Here's how the part is built. I have some questions about the finished solid (model axes, mm). A direction names the side the tool comes from. Round coordinates to 2 decimals unless told otherwise and drop trailing zeros. Write each loop counter-clockwise with the first axis right and the second up, starting at its lowest first coordinate (ties: lowest second). Pieces come first, ordered by that corner, then holes. Notation, with made-up numbers: (14, 8) - (70, 8) arc R17 cw to (70, 14) - close; hole circle Ø1 at (21.25, 1.5). An arc over 180 degrees is marked (long way). One line per question, with ' | ' between items. Start each with the question number.
(1) If I drill on L1, parallel to Z at x = -10.5, y = 4.25; L2, parallel to X at y = -1, z = 5.25; L3, parallel to Y at x = 1.5, z = 4, over which ranges is the centre line in solid material (lowest first)?
(2) For faces 1 (the flat face through (5, -10, 2)), 2 (the cylindrical face through (0.54, -2.44, 3.55)), which set-ups out of +Z, -Z, +X, -X, +Y, -Y let a thin tool reach every point of the face, with its end or its side?
(3) Will these pins go through, and if not, where does the flat tip stop? pin 1 (1 mm diameter, centred on x = -3.5, z = 1, fed in from +Y); pin 2 (1 mm diameter, centred on x = 1, z = 3.5, fed in from -Y); pin 3 (2 mm diameter, centred on x = 7, y = 0, fed in from +Z); pin 4 (1 mm diameter, centred on y = 0.5, z = 4, fed in from -X).
(4) Thinking about a two-plate mould opening in X: for faces 3 (the cylindrical face through (-11.99, 0.53, 6.19)), 4 (the flat face through (-3, 0, 0)), 5 (the cylindrical face through (5.75, 0.05, 3.65)), which applies, pulls with the +X half, pulls with the -X half, needs draft (parallel to the pull), parting line crosses it, or undercut?
(5) Imagine slicing it at A-A (z = 3.25). Write out the boundary of the cut face in (x, y), plus the area to 3 significant figures.
from build123d import *

# Parameters (mm, degrees)
SKETCH_1_R          = 12
EXTRUDE_1_DEPTH     = 2
SKETCH_2_R          = 11
EXTRUDE_2_DEPTH     = 3.2
SKETCH_3_R          = 12
EXTRUDE_3_DEPTH     = 2
SKETCH_4_R          = 2.5
CUT_EXTRUDE_1_DEPTH = 30
SKETCH_3D_1_R       = 1.597010155
M3X0_5_1_D          = 2.5
M3X0_5_1_DEPTH      = 8.5
M3X0_5_1_TIP        = 0.751075774


with BuildPart() as part:
    # ｽｹｯﾁ1 → ﾎﾞｽ - 押し出し1 (new body)
    with BuildSketch(Plane.XY):
        Circle(SKETCH_1_R)
    extrude(amount=EXTRUDE_1_DEPTH)

    # ｽｹｯﾁ2 → ﾎﾞｽ - 押し出し2 (add)
    with BuildSketch(Plane.XY.offset(2)):
        Circle(SKETCH_2_R)
    extrude(amount=EXTRUDE_2_DEPTH)

    # ｽｹｯﾁ3 → ﾎﾞｽ - 押し出し3 (add)
    with BuildSketch(Plane.XY.offset(5.2)):
        Circle(SKETCH_3_R)
    extrude(amount=EXTRUDE_3_DEPTH)

    # ｽｹｯﾁ4 → ｶｯﾄ - 押し出し1 (cut)
    with BuildSketch(Plane(origin=(0, 0, 0), x_dir=(-1, 0, 0), z_dir=(0, 0, -1))):
        Circle(SKETCH_4_R)
    extrude(amount=-CUT_EXTRUDE_1_DEPTH, mode=Mode.SUBTRACT)

    # ｶｯﾄ - ｽｲｰﾌﾟ1: sweep along a curve in space
    with BuildLine() as sweep_1_path:
        ThreePointArc((11, 0, 5.2), (7.778174593, 7.778174593, 5.2), (0, 11, 5.2))
        ThreePointArc((0, 11, 5.2), (-7.778174593, 7.778174593, 5.2), (-11, 0, 5.2))
        ThreePointArc((-11, 0, 5.2), (-7.778174593, -7.778174593, 5.2), (0, -11, 5.2))
        ThreePointArc((0, -11, 5.2), (7.778174593, -7.778174593, 5.2), (11, 0, 5.2))
    # Sketch 3D_1 → ｶｯﾄ - ｽｲｰﾌﾟ1 (sweep, cut)
    with BuildSketch(Plane(origin=(11, 0, 5.2), x_dir=(0, 0, -1), z_dir=(0, -1, 0))):
        with Locations((1.602989845, 0)):
            Circle(SKETCH_3D_1_R)
    sweep(path=sweep_1_path.line, mode=Mode.SUBTRACT)

    # M3x0.5 ねじ穴1
    with Locations(Plane(origin=(7, 0, 0), x_dir=(-1, 0, 0), z_dir=(0, 0, -1))):
        with Locations((0, 0)):
            Hole(M3X0_5_1_D / 2, depth=M3X0_5_1_DEPTH)
            with Locations((0, 0, -(M3X0_5_1_DEPTH + M3X0_5_1_TIP / 2))):  # 118° drill point
                Cone(0, M3X0_5_1_D / 2, M3X0_5_1_TIP, mode=Mode.SUBTRACT)


solid = part.part
Check sheet entries:
1) L1: 0 to 2, 5.2 to 7.2 | L2: -11.96 to -2.29, 2.29 to 6.25, 7.75 to 11.96 | L3: -9.33 to -2, 2 to 9.33
2) face 1: none | face 2: +Z, -Z
3) pin 1: y = 11.62 | pin 2: y = -9.47 | pin 3: through | pin 4: x = -9.67
4) face 3: parting line crosses it | face 4: needs draft | face 5: undercut
5) outline: circle Ø18.88 at (0, 0); hole circle Ø5 at (0, 0); hole circle Ø2.5 at (7, 0) | area: 255 mm^2
